Drawing for the job (mm, zero at the part's lowest x, y, z). Give positions to 0.01 mm unless a question says otherwise; leave off trailing zeros. Loops run counter-clockwise (first coordinate to the right, second up) from the corner with the lowest first, then second, coordinate; pieces in that order, holes last. Notation, with made-up numbers: (-5, 82.5) - (25, 82.5) arc R19 cw to (25, 89.5) - close; hole circle Ø4 at (13, -25). An arc over 180 degrees is marked (long way). Return JSON: item names as keys, results as strings. Group by question number.
1) Mould opens along Y. For the marked faces 1, 2 and 3 say: released by +Y, released by -Y, zero draft, split by the parting line, or undercut.
2) Slice it at D-D (z = 7.5). List the corners of the cut face in (x, y).
3) Slice it at C-C (z = 6). List the corners of the cut face in (x, y), and give its area (3 significant figures).
4) Drop flat-ended pins along their axis: pin 1 (1 mm diameter, centred on x = 8.5, z = 3.5, fed in from -Y); pin 2 (6 mm diameter, centred on x = 2, z = 5, fed in from -Y) (1 decimal). Give the stop position or say it passes through.
5) Drill centre lines: probe 1 along Y at (x, z) = (6.35, 10); probe 2 along Y at (x, z) = (5.25, 6.75) (1 decimal); probe 3 along Z at (x, y) = (7.5, 6.25). Where is each one in solid material? Low to high. Write a range as from..to.
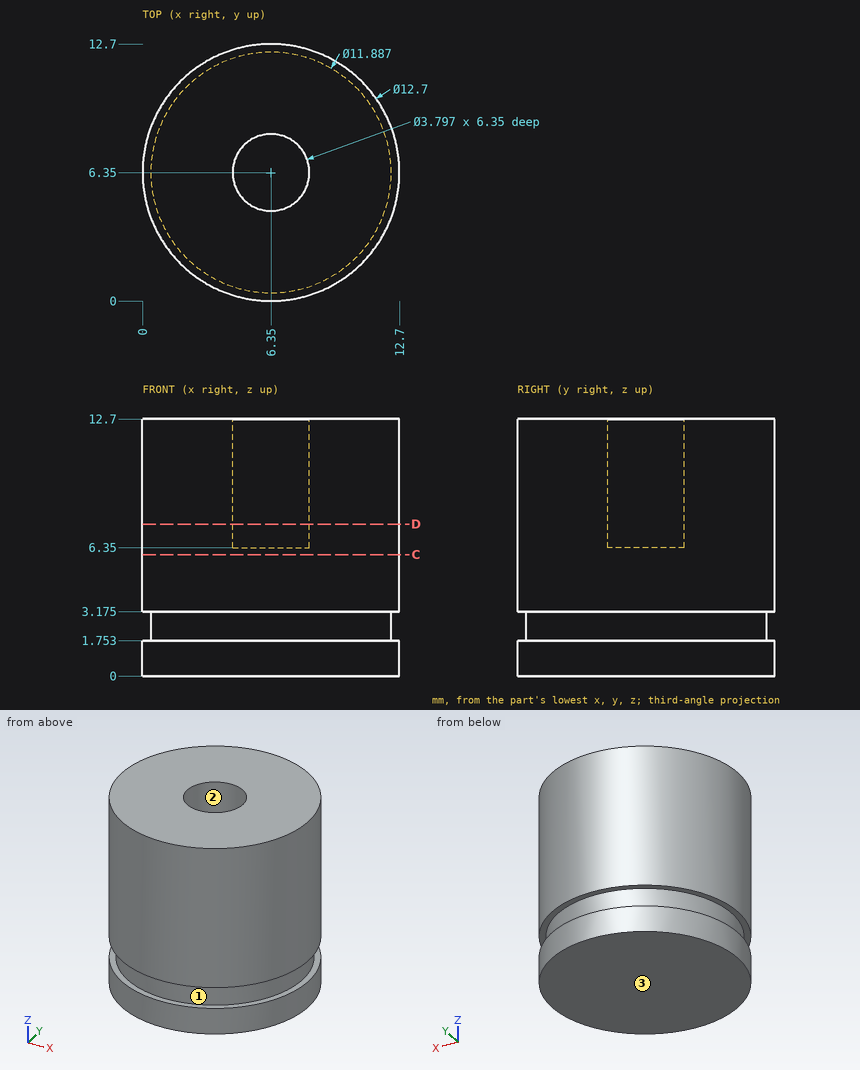
Results:
{
 "1": {"face 1": "split by the parting line", "face 2": "undercut", "face 3": "zero draft"},
 "2": {"outline": "circle Ø12.7 at (6.35, 6.35); hole circle Ø3.8 at (6.35, 6.35)"},
 "3": {"outline": "circle Ø12.7 at (6.35, 6.35)", "area": "127 mm2"},
 "4": {"pin 1": "y = 0.22", "pin 2": "y = 0.1"},
 "5": {"probe 1": "0..4.45, 8.25..12.7", "probe 2": "0.1..4.8, 7.9..12.6", "probe 3": "0..6.35"}
}
